from build123d import *

# Parameters (mm, degrees)
F0_W     = 106
F0_H     = 89
F1_DEPTH = 1
F0_W_2   = 20
F0_H_2   = 1
F0_W_3   = 1
F0_H_3   = 20
F2_DEPTH = 3
F3_DEPTH = 2
F4_R     = 3
F5_R     = 5
F6_SIZE2 = 2.4
F6_SIZE  = 2.4
F7_R     = 1.99999


# Not quite as in the source:
# - a fillet or chamfer is up to 0.001 mm smaller than in the source, because OpenCascade refuses the exact size


with BuildPart() as f1:
    # F0 (on Top) → F1 (new body)
    with BuildSketch(Plane.XY):
        Rectangle(F0_W, F0_H)
        Polygon((-47, 10), (-47, 38.5), (-10, 38.5), (-10, 39.5), (10, 39.5), (10, 38.5), (47, 38.5), (47, 10), (48, 10), (48, -10), (47, -10), (47, -38.5), (10, -38.5), (10, -39.5), (-10, -39.5), (-10, -38.5), (-47, -38.5), (-47, -10), (-48, -10), (-48, 10), align=None, mode=Mode.SUBTRACT)
    extrude(amount=F1_DEPTH)

    # F0 (on Top) → F2 (join)
    with BuildSketch(Plane.XY):
        with Locations((0, 39)):
            Rectangle(F0_W_2, F0_H_2)
        with Locations((-47.5, 0)):
            Rectangle(F0_W_3, F0_H_3)
        with Locations((47.5, 0)):
            Rectangle(F0_W_3, F0_H_3)
        with Locations((0, -39)):
            Rectangle(F0_W_2, F0_H_2)
    extrude(amount=F2_DEPTH)

    # F0 (on Top) → F3 (join)
    with BuildSketch(Plane.XY):
        Rectangle(F0_W, F0_H)
        Polygon((-47, 10), (-47, 38.5), (-10, 38.5), (-10, 39.5), (10, 39.5), (10, 38.5), (47, 38.5), (47, 10), (48, 10), (48, -10), (47, -10), (47, -38.5), (10, -38.5), (10, -39.5), (-10, -39.5), (-10, -38.5), (-47, -38.5), (-47, -10), (-48, -10), (-48, 10), align=None, mode=Mode.SUBTRACT)
        with Locations((0, 39)):
            Rectangle(F0_W_2, F0_H_2)
        with Locations((47.5, 0)):
            Rectangle(F0_W_3, F0_H_3)
        with Locations((-47.5, 0)):
            Rectangle(F0_W_3, F0_H_3)
        with Locations((0, -39)):
            Rectangle(F0_W_2, F0_H_2)
    extrude(amount=-F3_DEPTH)

    # F4
    f4_edges = [f1.edges().sort_by_distance(p)[0] for p in [
        (47, 38.5, -0.5),
        (47, -38.5, -0.5),
        (-47, 38.5, -0.5),
        (-47, -38.5, -0.5),
    ]]
    fillet(f4_edges, radius=F4_R)

    # F5
    f5_edges = [f1.edges().sort_by_distance(p)[0] for p in [
        (-53, -44.5, -0.5),
        (53, -44.5, -0.5),
        (-53, 44.5, -0.5),
        (53, 44.5, -0.5),
    ]]
    fillet(f5_edges, radius=F5_R)

    # F6
    f6_edges = [f1.edges().sort_by_distance(p)[0] for p in [
        (0, -44.5, -2),
    ]]
    chamfer(f6_edges, length=F6_SIZE, length2=F6_SIZE2)

    # F7 (radius 2 in the source; OpenCascade refuses exactly that, so slightly less here)
    f7_edges = [f1.edges().sort_by_distance(p)[0] for p in [
        (10, -39, 3),
        (-10, -39, 3),
        (-47.5, -10, 3),
        (-47.5, 10, 3),
        (-10, 39, 3),
        (10, 39, 3),
        (47.5, 10, 3),
        (47.5, -10, 3),
    ]]
    fillet(f7_edges, radius=F7_R)


solid = f1.part
Build history of the part. All positions in model axes, mm. A direction names the side the tool comes from. Coordinates: 2 decimals unless noted, no trailing zeros. Order: outer loops, then holes, each group sorted by start corner. A loop starts at its lowest first (then second) coordinate and runs counter-clockwise, first axis right, second up. Notation, with made-up numbers: (-17.5, 75) - (27.5, 75) arc R29 ccw to (27.5, 98) - close; hole circle Ø10 at (73.5, 71). An arc over 180 degrees is marked (long way). Write each question's results on one line, items separated by ' | '. Start each with the question number.
Item 1: Band-saw the part on B-B on y = 5.5. Write the cut outline in (x, z), and give its area (3 significant figures).
Item 2: Band-saw the part on A-A on x = -4. Write the cut outline in (y, z), and give its area (3 significant figures).
Item 3: Band-saw the part on C-C on z = -1.05. Write the cut outline in (x, y).
Item 4: Wall check: probe 1 along X at (y, z) = (-8, 2.1); probe 2 along Y at (x, z) = (-22, 0.85); probe 3 along X at (y, z) = (-40, 0.7). Give the ranges that are in metal, low to high. Write a range as [from, to].
Item 5: Mould opens along Y. For faces 3 (the face through (46.14, -37.6, -0.48)), 4 (the face through (51.8, -0.6, -0.8)), 5 (the face through (-51.57, -43, 0.7)), 6 (the face through (-50.459, 42.014, -1.083)) say: released by +Y, released by -Y, zero draft, split by the parting line, or undercut.
Item 6: Flat gauge pins, fed straight in: pin 1 (2 mm diameter, centred on y = 0.5, z = 2.5, fed in from -X); pin 2 (1.6 mm diameter, centred on x = -1, z = 2, fed in from +Y); pin 3 (1.5 mm diameter, centred on y = 5.5, z = -1, fed in from +X). Where does each tip first touch, or does it go through?
Item 7: Band-saw the part on D-D on x = -41.5. Write the cut outline in (y, z).
Item 8: Tool access for faces 1 (the face through (46.1, 37.64, -0.48)), 2 (the face through (-51.57, 43, 0.7)): list every direction of +Z, -Z, +X, -X, +Y, -Y with a clear straight run to the whole face (end or side of a thin tool).
Numbers:
1) outline: (-53, 0.4) - (-50.6, -2) - (-47, -2) - (-47, 3) - (-48, 3) - (-48, 1) - (-53, 1) - close; (47, -2) - (50.6, -2) - (53, 0.4) - (53, 1) - (48, 1) - (48, 3) - (47, 3) - close | area: 34.2 mm^2
2) outline: (-44.5, 0.4) - (-42.1, -2) - (-38.5, -2) - (-38.5, 3) - (-39.5, 3) - (-39.5, 1) - (-44.5, 1) - close; (38.5, -2) - (42.1, -2) - (44.5, 0.4) - (44.5, 1) - (39.5, 1) - (39.5, 3) - (38.5, 3) - close | area: 34.2 mm^2
3) outline: (-51.55, -39.5) arc R3.55 ccw to (-48, -43.05) - (48, -43.05) arc R3.55 ccw to (51.55, -39.5) - (51.55, 39.5) arc R3.55 ccw to (48, 43.05) - (-48, 43.05) arc R3.55 ccw to (-51.55, 39.5) - close; hole (-47, -35.5) arc R3 ccw to (-44, -38.5) - (44, -38.5) arc R3 ccw to (47, -35.5) - (47, 35.5) arc R3 ccw to (44, 38.5) - (-44, 38.5) arc R3 ccw to (-47, 35.5) - close
4) probe 1: [-48, -47], [47, 48] | probe 2: [-44.5, -38.5], [38.5, 44.5] | probe 3: [-52.97, 52.97]
5) face 3: undercut | face 4: zero draft | face 5: released by -Y | face 6: released by +Y
6) pin 1: x = -48 | pin 2: y = 39.5 | pin 3: x = 52.35
7) outline: (-44.5, 0.4) - (-42.1, -2) - (-38.5, -2) - (-38.5, 1) - (-44.5, 1) - close; (38.5, -2) - (42.1, -2) - (44.5, 0.4) - (44.5, 1) - (38.5, 1) - close
8) face 1: +Z, -Z | face 2: +Z, -Z, -X, +Y
